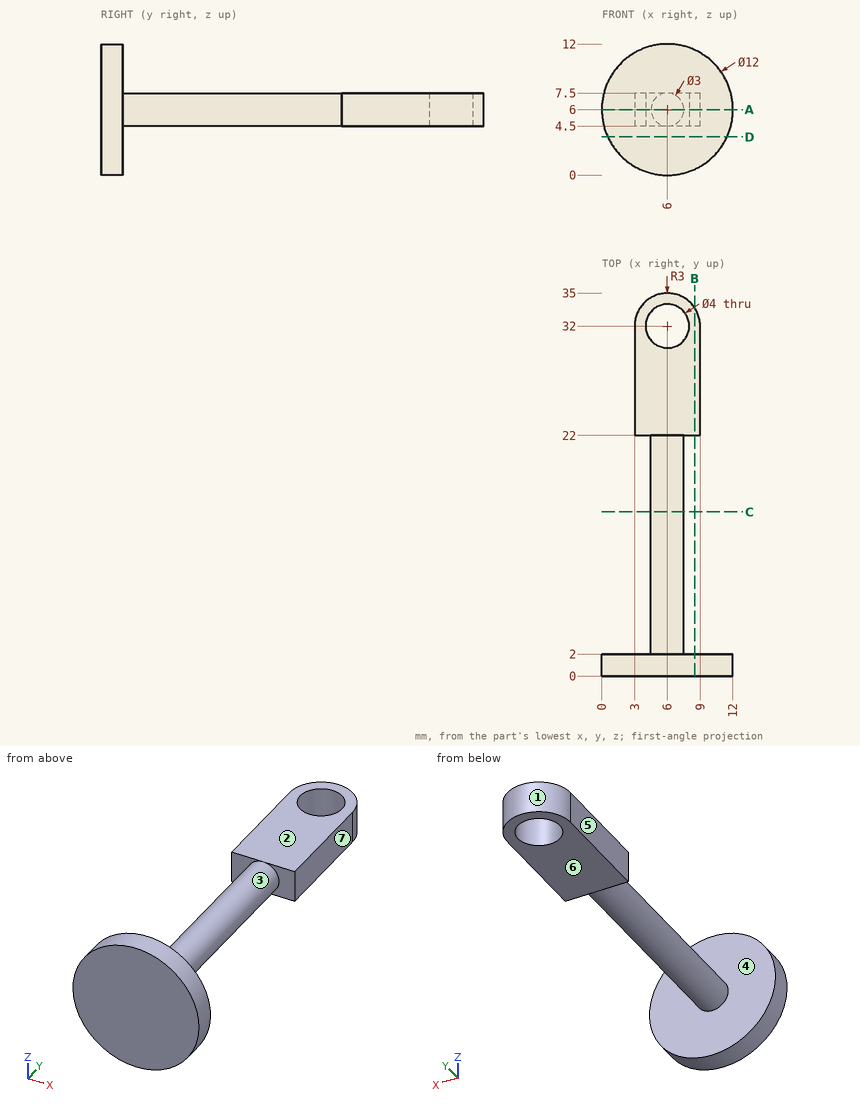
Source: three-view drawing plus pictorial views. Frame: mm from the lowest corner of the part. A direction names the side the tool comes from. Round coordinates to 2 decimals unless told otherwise and drop trailing zeros. Order: outer loops, then holes, each group sorted by start corner. A loop starts at its lowest first (then second) coordinate and runs counter-clockwise, first axis right, second up. Notation, with made-up numbers: (31, 74) -> (85, 74) arc R9 cw to (85, 88) -> close; hole circle Ø10 at (-2.5, 21). An arc over 180 degrees is marked (long way). Use one line per item in the form item = value. Start each with the question number.
1. Cut plane B-B (x = 8.5). Return the cut outline in (y, z).
2. Pin query (flat end, axial travel): pin 1 Ø6 at (x, z) = (9.5, 10.5) entering from +Y; pin 2 Ø3 at (x, y) = (7, 27) entering from -Z; pin 3 Ø1.5 at (y, z) = (25, 5.5) entering from +X. Return the tip coordinate at first contact, or that it passes through.
3. Cut plane A-A (z = 6). Return the cut outline in (x, y).
4. Reachability of the marked faces 4, 5, 6 and 7 from +Z, -Z, +X, -X, +Y, -Y: full face, straight path, thin tool, end or side. Return the list, or none.
5. Cut plane D-D (z = 3.5). Return the cut outline in (x, y).
6. Cut plane C-C (y = 15). Return the cut outline in (x, z), then the cut area to 3 significant figures.
7. Draft query along Y for the marked faces 1, 2 and 3. Return one class per face: pulls with the +Y half, pulls with the -Y half, needs draft (parallel to the pull), parting line crosses it, or undercut.
8. Line query: probe 1 along Y at (x, z) = (6, 5.95); probe 2 along Y at (x, z) = (6, 2.75); probe 3 along Z at (x, y) = (5, 25.5). Output: solid intervals per line, ascending.
Solution:
q1.outline = (0, 0.55) -> (2, 0.55) -> (2, 11.45) -> (0, 11.45) -> close; (22, 4.5) -> (33.66, 4.5) -> (33.66, 7.5) -> (22, 7.5) -> close
q2.pin_1 = 2
q2.pin_2 = 4.5
q2.pin_3 = 9
q3.outline = (0, 0) -> (12, 0) -> (12, 2) -> (7.5, 2) -> (7.5, 22) -> (9, 22) -> (9, 32) arc R3 ccw to (3, 32) -> (3, 22) -> (4.5, 22) -> (4.5, 2) -> (0, 2) -> close; hole circle Ø4 at (6, 32)
q4.face_4 = none
q4.face_5 = +Z, -Z, -X, +Y
q4.face_6 = -Z, +X, -X, +Y
q4.face_7 = +Z, -Z, +X, +Y
q5.outline = (0.55, 0) -> (11.45, 0) -> (11.45, 2) -> (0.55, 2) -> close
q6.outline = circle Ø3 at (6, 6)
q6.area = 7.07 mm^2
q7.face_1 = pulls with the +Y half
q7.face_2 = needs draft
q7.face_3 = undercut
q8.probe_1 = 0 to 30, 34 to 35
q8.probe_2 = 0 to 2
q8.probe_3 = 4.5 to 7.5
